from build123d import *

# Parameters (mm, degrees)
BOSS_EXTRUDE1_DEPTH = 27


with BuildPart() as part:
    # Sketch2 → Boss-Extrude1 (new body)
    with BuildSketch(Plane(origin=(0, 0, 0), x_dir=(1, 0, 0), z_dir=(0, 1, 0))):
        with BuildLine():
            Line((1.949489743, 2.280238966), (25.332175645, 15.780238966))
            ThreePointArc((25.332175645, 15.780238966), (34.918685713, 16.839438194), (42.188333234, 10.501039089))
            ThreePointArc((42.188333234, 10.501039089), (34.951918852, 15.366431786), (26.332175645, 14.048188159))
            Line((26.332175645, 14.048188159), (2.949489743, 0.548188159))
            ThreePointArc((2.949489743, 0.548188159), (2.987345747, 0.275255129), (3, 0))
            ThreePointArc((3, 0), (2.987345747, -0.275255129), (2.949489743, -0.548188159))
            Line((2.949489743, -0.548188159), (26.332175645, -14.048188159))
            ThreePointArc((26.332175645, -14.048188159), (32.042724118, -21.820749797), (30.188333234, -31.285648779))
            ThreePointArc((30.188333234, -31.285648779), (30.783679718, -22.586033743), (25.332175645, -15.780238966))
            Line((25.332175645, -15.780238966), (1.949489743, -2.280238966))
            ThreePointArc((1.949489743, -2.280238966), (1.732050808, -2.449489743), (1.5, -2.598076211))
            ThreePointArc((1.5, -2.598076211), (1.25529494, -2.724744871), (1, -2.828427125))
            Line((1, -2.828427125), (1, -29.828427125))
            ThreePointArc((1, -29.828427125), (-2.875961595, -38.660187991), (-12, -41.786687868))
            ThreePointArc((-12, -41.786687868), (-4.168239134, -37.952465529), (-1, -29.828427125))
            Line((-1, -29.828427125), (-1, -2.828427125))
            ThreePointArc((-1, -2.828427125), (-1.25529494, -2.724744871), (-1.5, -2.598076211))
            ThreePointArc((-1.5, -2.598076211), (-1.732050808, -2.449489743), (-1.949489743, -2.280238966))
            Line((-1.949489743, -2.280238966), (-25.332175645, -15.780238966))
            ThreePointArc((-25.332175645, -15.780238966), (-34.918685713, -16.839438194), (-42.188333234, -10.501039089))
            ThreePointArc((-42.188333234, -10.501039089), (-34.951918852, -15.366431786), (-26.332175645, -14.048188159))
            Line((-26.332175645, -14.048188159), (-2.949489743, -0.548188159))
            ThreePointArc((-2.949489743, -0.548188159), (-2.987345747, -0.275255129), (-3, 0))
            ThreePointArc((-3, 0), (-2.987345747, 0.275255129), (-2.949489743, 0.548188159))
            Line((-2.949489743, 0.548188159), (-26.332175645, 14.048188159))
            ThreePointArc((-26.332175645, 14.048188159), (-32.042724118, 21.820749797), (-30.188333234, 31.285648779))
            ThreePointArc((-30.188333234, 31.285648779), (-30.783679718, 22.586033743), (-25.332175645, 15.780238966))
            Line((-25.332175645, 15.780238966), (-1.949489743, 2.280238966))
            ThreePointArc((-1.949489743, 2.280238966), (-1.732050808, 2.449489743), (-1.5, 2.598076211))
            ThreePointArc((-1.5, 2.598076211), (-1.25529494, 2.724744871), (-1, 2.828427125))
            Line((-1, 2.828427125), (-1, 29.828427125))
            ThreePointArc((-1, 29.828427125), (2.875961595, 38.660187991), (12, 41.786687868))
            ThreePointArc((12, 41.786687868), (4.168239134, 37.952465529), (1, 29.828427125))
            Line((1, 29.828427125), (1, 2.828427125))
            ThreePointArc((1, 2.828427125), (1.25529494, 2.724744871), (1.5, 2.598076211))
            ThreePointArc((1.5, 2.598076211), (1.732050808, 2.449489743), (1.949489743, 2.280238966))
        make_face()
    extrude(amount=BOSS_EXTRUDE1_DEPTH)


solid = part.part
Check sheet for the modelled part. Datum: model origin and axes. Units: mm. A direction names the side the tool comes from. Round coordinates to 2 decimals unless told otherwise and drop trailing zeros. Write each loop counter-clockwise with the first axis right and the second up, starting at its lowest first coordinate (ties: lowest second). Pieces come first, ordered by that corner, then holes. Notation, with made-up numbers: (24.5, 51) -> (57.5, 51) arc R20 cw to (57.5, 84) -> close; hole circle Ø1 at (33.5, -12). An arc over 180 degrees is marked (long way). Answer as CSV lines item,"result". Start each with the question number.
1) Section check D-D on z = 35.5. Enter the section's corners in (x, y).
2) Material ranges on line 1 (X direction, y = 14.75, z = 7.5); line 2 (Z direction, x = 9.5, y = 18.5); line 3 (Z direction, x = -5, y = 22.75), recorded low to high. Write a range as from..to.
3) Tool access check on faces 4 (the flat face through (1, 13, 16)), 5 (the cylindrical face through (-4.25, 13.31, 38.04)), 6 (the cylindrical face through (-30.82, 13.31, -22.71)). Record the directions out of +Z, -Z, +X, -X, +Y, -Y that give a thin tool (end or side, any length) a straight path to the whole face; none if there is none.
4) Section check B-B on x = 17.5. Enter the section's corners in (y, z), and give its area (3 significant figures).
5) Release check for a two-part mould opening along Z. For faces 1 (the flat face through (-1, 13, 17)), 2 (the flat face through (0, 0, 0)), 3 (the flat face through (13.8, 13.31, 9.12)) record: pulls with the +Z half, pulls with the -Z half, needs draft (parallel to the pull), parting line crosses it, or undercut.
6) Section check C-C on z = -21. Enter the section's corners in (x, y).
7) Section check A-A on z = -8.5. Enter the section's corners in (x, y), and give its area (3 significant figures).
8) Go/stop test with flat-tipped pins: P1, Ø10, axis at y = 18.5, z = -26, coming from the -X side; P2, Ø2, axis at y = 6, z = -29, coming from the -X side; P3, Ø8, axis at x = 3, z = 32, coming from the +Y side; P4, Ø8, axis at y = 16, z = 15.5, coming from the +X side. Record where each tip stops, or that it passes through.
Found:
1,outline,"(-2.42, 0) -> (-0.42, 0) -> (-0.42, 27) -> (-2.42, 27) -> close"
2,line 1,"x = -14.99..-10.99, -1..1, 10.99..14.99"
2,line 2,"z = -41.73..-41.31, -6.64..-4.33, 4.33..6.64"
2,line 3,"z = -4.04..-1.73, 1.73..4.04, 38.77..40.22"
3,face 4,"+Z, +Y, -Y"
3,face 5,"-X, +Y, -Y"
3,face 6,"+Y, -Y"
4,outline,"(0, -11.26) -> (27, -11.26) -> (27, -8.95) -> (0, -8.95) -> close; (0, 8.95) -> (27, 8.95) -> (27, 11.26) -> (0, 11.26) -> close"
4,area,"125 mm^2"
5,face 1,"undercut"
5,face 2,"needs draft"
5,face 3,"pulls with the +Z half"
6,outline,"(-31.83, 0) -> (-30.16, 0) -> (-30.16, 27) -> (-31.83, 27) -> close; (-1, 0) -> (1, 0) -> (1, 27) -> (-1, 27) -> close"
7,outline,"(-16.72, 0) -> (-12.72, 0) -> (-12.72, 27) -> (-16.72, 27) -> close; (-1, 0) -> (1, 0) -> (1, 27) -> (-1, 27) -> close; (12.72, 0) -> (16.72, 0) -> (16.72, 27) -> (12.72, 27) -> close"
7,area,"270 mm^2"
8,P1,"stops at x = -32.33"
8,P2,"stops at x = -31.79"
8,P3,"stops at y = 27"
8,P4,"stops at x = 31.27"
